Work out the finished part from the listing and answer in its coordinate system (mm). Coordinates: 2 decimals unless noted, no trailing zeros. Loops run counter-clockwise (first coordinate to the right, second up) from the corner with the lowest first, then second, coordinate; pieces in that order, holes last. Notation, with made-up numbers: (-19.75, -37.75) -> (-6.75, -37.75) arc R17 ccw to (-6.75, -20.75) -> close; hole circle Ø5 at (0.5, 70.5). An arc over 180 degrees is marked (long way). Use a Markdown table: item, result. Add a question column.
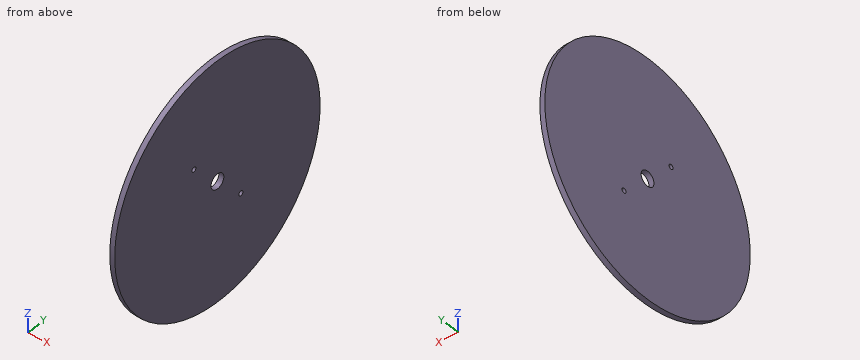
```python
from build123d import *

# Parameters (mm, degrees)
F0_R     = 76.2
F0_R_2   = 4.7625
F1_DEPTH = 3.175
F2_R     = 1.5875
F3_DEPTH = 3.176
F4_R     = 1.4986
F5_DEPTH = 25.4


with BuildPart() as f1:
    # F0 (on Right) → F1 (new body)
    with BuildSketch(Plane.YZ):
        Circle(F0_R)
        Circle(F0_R_2, mode=Mode.SUBTRACT)
    extrude(amount=F1_DEPTH)

    # F2 (on face) → F3 (cut, through all)
    with BuildSketch(Plane.YZ.offset(3.175)):
        Circle(F2_R)
    extrude(amount=-F3_DEPTH, mode=Mode.SUBTRACT)

    # F4 (on face) → F5 (cut)
    with BuildSketch(Plane.YZ.offset(3.175)):
        with Locations((-17.420961, 18.484321)):
            Circle(F4_R)
        with Locations((17.420961, -18.484321)):
            Circle(F4_R)
    extrude(amount=-F5_DEPTH, mode=Mode.SUBTRACT)


solid = f1.part
```
Item 1: Section A-A (z = 0) is taken. Determine the outline of the cut face in (x, y) (1 decimal), then the cut area to 3 significant figures.
Item 2: Section D-D (z = -60) is taken. Determine the outline of the cut face in (x, y) (3 decimals).
Item 3: Given pin 1 (1 mm diameter, centred on x = 1, y = -58, fed in from -Z); pin 2 (1 mm diameter, centred on x = 1.5, z = -34.5, fed in from +Y); pin 3 (2.5 mm diameter, centred on y = 17.42, z = -18.48, fed in from +X); pin 4 (3.5 mm diameter, centred on y = -17.42, z = 18.48, fed in from +X) (3 decimals), each flat-ended and moving along its own axis, determine where each tip first touches the part or whether it passes through.
Item 4: Find the intervals of material crossed by probe 1 along Z at (x, y) = (1.8, 0); probe 2 along Z at (x, y) = (2.75, 17.5); probe 3 along Y at (x, z) = (2.3, 17.5), in increasing order.
Item 5: Section C-C (x = 0.8) is taken. Determine the outline of the cut face in (y, z) (1 decimal), then the cut area to 3 significant figures.
Output:
| question | item | result |
|---|---|---|
| 1 | outline | (0, -76.2) -> (3.2, -76.2) -> (3.2, -4.8) -> (0, -4.8) -> close; (0, 4.8) -> (3.2, 4.8) -> (3.2, 76.2) -> (0, 76.2) -> close |
| 1 | area | 454 mm2 |
| 2 | outline | (0, -46.973) -> (3.175, -46.973) -> (3.175, 46.973) -> (0, 46.973) -> close |
| 3 | pin 1 | stops at z = -50 |
| 3 | pin 2 | stops at y = 68.19 |
| 3 | pin 3 | passes through |
| 3 | pin 4 | stops at x = 3.175 |
| 4 | probe 1 | z = -76.2 to -4.76, 4.76 to 76.2 |
| 4 | probe 2 | z = -74.16 to -19.98, -16.99 to 74.16 |
| 4 | probe 3 | y = -74.16 to -18.55, -16.29 to 74.16 |
| 5 | outline | circle Ø152.4 at (0, 0); hole circle Ø3 at (-17.4, 18.5); hole circle Ø9.5 at (0, 0); hole circle Ø3 at (17.4, -18.5) |
| 5 | area | 18,200 mm2 |
